Autodesk Inventor part; units mm, degrees
ref_plane "YZ Plane" through (0, 0, 0) normal (1, 0, 0) x (0, 1, 0)
ref_plane "XZ Plane" through (0, 0, 0) normal (0, 1, 0) x (-1, 0, 0)
ref_plane "XY Plane" through (0, 0, 0) normal (0, 0, 1) x (1, 0, 0)
sketch "Sketch1" plane through (0, 0, 0) normal (0, 0, 1) x (1, 0, 0)
  circle A0 centre (0, 0) radius 12.7
  circle A1 centre (0, 0) radius 44.45
  dimension "d0" = 25.4
  dimension "d1" = 88.9
extrude "Extrusion1" add sketch "Sketch1" along normal blind 6.35
sketch "Sketch2" plane through (0, 0, 0) normal (0, 0, -1) x (-1, 0, 0)
  circle A0 centre (0, 0) radius 19.05
  circle A1 centre (0, -19.05) radius 3.3782
  circle A2 centre (16.4978, -9.525) radius 3.3782
  circle A3 centre (16.4978, 9.525) radius 3.3782
  circle A4 centre (0, 19.05) radius 3.3782
  circle A5 centre (-16.4978, 9.525) radius 3.3782
  circle A6 centre (-16.4978, -9.525) radius 3.3782
  dimension "d4" = 38.1
  dimension "d5" = 6.7564
  dimension "d8" = 360
extrude "Extrusion2" cut sketch "Sketch2" against normal blind 6.35 contours A3 A0 | A0 A3 | A2 A0 | A0 A2 | A4 A0 | A0 A4 | A1 A0 | A0 A1 | A5 A0 | A0 A5 | A6 A0 | A0 A6
properties part number "AZUSASprocketSmall"
Input: part model. Units: mm. Frame: model coordinates. Coordinates: 2 decimals unless noted, no trailing zeros. Loops run counter-clockwise (first coordinate to the right, second up) from the corner with the lowest first, then second, coordinate; pieces in that order, holes last. Notation, with made-up numbers: M 85,72 L 118,72 A21 cw 118,79 Z; hole C -15.75,59 d7. An arc over 180 degrees is marked long. Use a Markdown table: item, result. Add a question column.
1) Pin query (flat end, axial travel): P1, Ø3, axis at y = -27.5, z = 5.5, coming from the +X side; P2, Ø6, axis at x = 0, y = 19.05, coming from the +Z side; P3, Ø1, axis at x = 35, z = 3.5, coming from the +Y side; P4, Ø8, axis at x = 16.5, y = 9.52, coming from the +Z side. Return the tip coordinate at first contact, or that it passes through.
2) Line query: L1, parallel to Y at x = 0, z = 4.75; L2, parallel to Y at x = -14, z = 2; L3, parallel to X at y = -11.5, z = 4. Output: solid intervals per line, ascending. Write a range as from..to.
3) Section A-A, the plane y = 0. Return the cut outline in (x, z), plus the area to 3 significant figures.
4) Section C-C, the plane z = 5.25. Return the cut outline in (x, y) (3 decimals), plus the area to 3 significant figures.
5) Draft query along X for faces 1 (the cylindrical face through (42.397, -13.352, 3.131)), 2 (the cylindrical face through (0.44, -15.7, 3.13)), 3 (the flat face through (9.3, -9.3, 0)). Return one class per face: +X half, -X half, draft (parallel to the pull), parting line (faces both ways), or undercut.
6) Section D-D, the plane y = 19.05. Return the cut outline in (x, z).
7) Section B-B, the plane x = 0. Return the cut outline in (y, z).
Answer below:
| question | item | result |
|---|---|---|
| 1 | P1 | x = 36.05 |
| 1 | P2 | through |
| 1 | P3 | y = 28.03 |
| 1 | P4 | z = 6.35 |
| 2 | L1 | -44.45..-22.43, -15.67..-12.7, 12.7..15.67, 22.43..44.45 |
| 2 | L2 | -42.19..-11.8, -7.25..7.25, 11.8..42.19 |
| 2 | L3 | -42.94..-19.24, -13.76..-5.39, 5.39..13.76, 19.24..42.94 |
| 3 | outline | M -44.45,0 L -12.7,0 L -12.7,6.35 L -44.45,6.35 Z; M 12.7,0 L 44.45,0 L 44.45,6.35 L 12.7,6.35 Z |
| 3 | area | 403 mm2 |
| 4 | outline | C 0,0 d88.9; hole C -16.498,-9.525 d6.756; hole C -16.498,9.525 d6.756; hole C 0,0 d25.4; hole C 0,-19.05 d6.756; hole C 0,19.05 d6.756; hole C 16.498,-9.525 d6.756; hole C 16.498,9.525 d6.756 |
| 4 | area | 5,490 mm2 |
| 5 | face 1 | parting line |
| 5 | face 2 | undercut |
| 5 | face 3 | draft |
| 6 | outline | M -40.16,0 L -3.38,0 L -3.38,6.35 L -40.16,6.35 Z; M 3.38,0 L 40.16,0 L 40.16,6.35 L 3.38,6.35 Z |
| 7 | outline | M -44.45,0 L -22.43,0 L -22.43,6.35 L -44.45,6.35 Z; M -15.67,0 L -12.7,0 L -12.7,6.35 L -15.67,6.35 Z; M 12.7,0 L 15.67,0 L 15.67,6.35 L 12.7,6.35 Z; M 22.43,0 L 44.45,0 L 44.45,6.35 L 22.43,6.35 Z |
